Build history of the part. All positions in model axes, mm. Face numbers are marked on the shaded views. Round coordinates to 2 decimals unless told otherwise and drop trailing zeros. Loops run counter-clockwise (first coordinate to the right, second up) from the corner with the lowest first, then second, coordinate; pieces in that order, holes last. Notation, with made-up numbers: (56, 65) - (98, 65) arc R26 ccw to (98, 82) - close; hole circle Ø1 at (-30.75, 77.5). An arc over 180 degrees is marked (long way). Put each result on its own line as item: value. Start each with the question number.
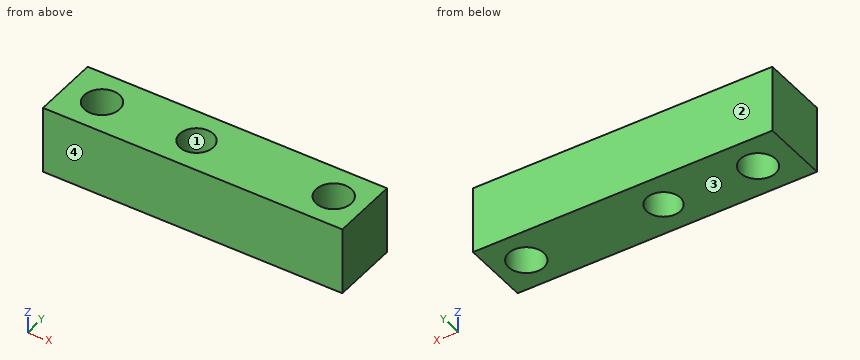
Autodesk Inventor part; units mm, degrees
ref_plane "YZ Plane" through (0, 0, 0) normal (1, 0, 0) x (0, 1, 0)
ref_plane "XZ Plane" through (0, 0, 0) normal (0, 1, 0) x (-1, 0, 0)
ref_plane "XY Plane" through (0, 0, 0) normal (0, 0, 1) x (1, 0, 0)
sketch "Sketch1" plane through (0, 0, 0) normal (0, 0, 1) x (1, 0, 0)
  line L0 (0, 0) -> (100, 0)
  line L1 (100, 0) -> (100, 20)
  line L2 (100, 20) -> (0, 20)
  line L3 (0, 20) -> (0, 0)
  dimension "d0" = 100
  dimension "d1" = 20
extrude "Extrusion1" add sketch "Sketch1" against normal blind 20
sketch "Sketch2" plane through (0, 0, 0) normal (0, 0, 1) x (1, 0, 0)
  line L0 (0, 0) -> (0, 20)
  circle A0 centre (44.5, 10) radius 5
  line L1 (0, 0) -> (100, 0)
  dimension "d5" = 10
  dimension "d24" = 44.5
  dimension "d25" = 10
sketch "Sketch3" plane through (0, 0, 0) normal (0, 0, 1) x (1, 0, 0)
  line L0 (0, 0) -> (0, 20)
  line L1 (100, 20) -> (100, 0)
  line L2 (100, 10) -> (85.3, 10)
  circle A0 centre (85.3, 10) radius 5.25
  dimension "d8" = 14.7
  dimension "d9" = 10.5
extrude "Extrusion2" cut sketch "Sketch3" against normal blind 20
extrude "Extrusion3" cut sketch "Sketch2" against normal blind 20
sketch "Sketch4" plane through (0, 0, 0) normal (0, 0, 1) x (1, 0, 0)
  line L0 (0, 20) -> (0, 0)
  circle A0 centre (16.4, 10) radius 5.25
  circle A1 centre (44.5, 10) radius 5
  line L1 (0, 0) -> (100, 0)
  dimension "d15" = 10.5
  dimension "d27" = 10
  dimension "d29" = 16.4
extrude "Extrusion4" cut sketch "Sketch4" against normal blind 20 contours A0
sketch "Sketch5" plane through (0, 0, 0) normal (0, 0, 1) x (1, 0, 0)
  point P0 (0, 0)
sketch "Sketch6" plane through (100, 0, 0) normal (1, 0, 0) x (0, 0, -1)
  line L0 (0, 0) -> (20, 0)
  line L1 (20, 0) -> (20, 20)
  line L2 (0, 0) -> (20, 0)
  line L3 (20, 0) -> (20, 20)
  line L4 (20, 20) -> (0, 20)
  line L5 (0, 20) -> (0, 0)
extrude "Extrusion5" cut sketch "Sketch6" against normal blind 5.5
sketch "Sketch7" plane through (0, 0, 0) normal (-1, 0, 0) x (0, 0, 1)
  line L0 (-20, 0) -> (-20, 20)
  line L1 (0, 20) -> (-20, 20)
  line L2 (-20, 0) -> (0, 0)
  line L3 (0, 0) -> (0, 20)
  line L4 (0, 20) -> (-20, 20)
  line L5 (-20, 20) -> (-20, 0)
extrude "Extrusion6" cut sketch "Sketch7" against normal blind 5.5
thread "Thread1"
properties part number "block"
1) Drill centre lines: line 1 (Y direction, x = 16.4, z = -10.5); line 2 (X direction, y = 8.75, z = -3.75); line 3 (X direction, y = 11.5, z = -3.75). Where is each one in solid material? Low to high. Write a range as [from, to].
2) Slice it at C-C, the plane y = 10. Write the cut outline in (x, z), and give its area (3 significant figures).
3) Slice it at B-B, the plane z = -13.25. Write the cut outline in (x, y), and give its area (3 significant figures).
4) Pull direction Y, two halves, no side cores. Call the marked faces 1, 2, 3 and 4: pulls with the +Y half, pulls with the -Y half, needs draft (parallel to the pull), parting line crosses it, or undercut.
5) Drop flat-ended pins along their axis: pin 1 Ø6.5 at (x, y) = (85.3, 10) entering from -Z; pin 2 Ø4 at (x, y) = (85.5, 5.5) entering from -Z. Give the stop position or say it passes through.
6) Slice it at D-D, the plane x = 85. Write the cut outline in (y, z).
7) Slice it at A-A, the plane x = 44.5. Write the cut outline in (y, z).
Taken from the geometry:
1. line 1: y = [0, 4.75], [15.25, 20]
1. line 2: x = [5.5, 11.3], [21.5, 39.66], [49.34, 80.2], [90.4, 94.5]
1. line 3: x = [5.5, 11.37], [21.43, 39.73], [49.27, 80.27], [90.33, 94.5]
2. outline: (5.5, -20) - (11.15, -20) - (11.15, 0) - (5.5, 0) - close; (21.65, -20) - (39.5, -20) - (39.5, 0) - (21.65, 0) - close; (49.5, -20) - (80.05, -20) - (80.05, 0) - (49.5, 0) - close; (90.55, -20) - (94.5, -20) - (94.5, 0) - (90.55, 0) - close
2. area: 1,160 mm2
3. outline: (5.5, 0) - (94.5, 0) - (94.5, 20) - (5.5, 20) - close; hole circle Ø10.5 at (16.4, 10); hole circle Ø10 at (44.5, 10); hole circle Ø10.5 at (85.3, 10)
3. area: 1,530 mm2
4. face 1: undercut
4. face 2: pulls with the +Y half
4. face 3: needs draft
4. face 4: pulls with the -Y half
5. pin 1: passes through
5. pin 2: stops at z = -20
6. outline: (0, -20) - (4.76, -20) - (4.76, 0) - (0, 0) - close; (15.24, -20) - (20, -20) - (20, 0) - (15.24, 0) - close
7. outline: (0, -20) - (5, -20) - (5, 0) - (0, 0) - close; (15, -20) - (20, -20) - (20, 0) - (15, 0) - close
